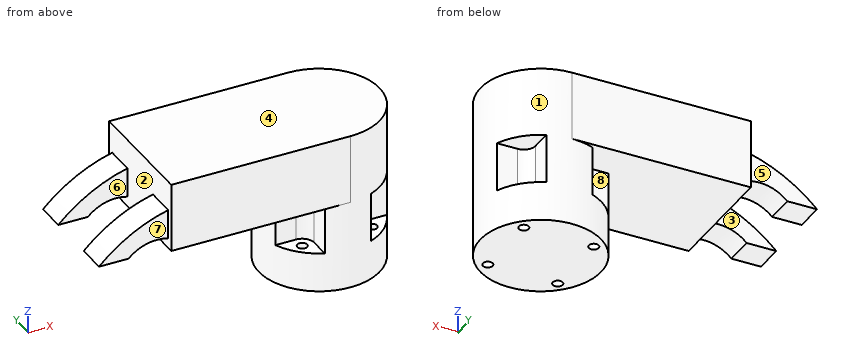
from build123d import *

# Parameters (mm, degrees)
SKETCH1_R                            = 30.5
BOSS_EXTRUDE1_DEPTH                  = 80
CUT_EXTRUDE1_REACH                   = 142.887
CUT_EXTRUDE1_START                   = -50
SKETCH2_R                            = 2.5
SKETCH7_W                            = 35
SKETCH7_H                            = 61
BOSS_EXTRUDE4_DEPTH                  = 60
BOSS_EXTRUDE4_DIRECTION_2_REACH      = 107.125
BOSS_EXTRUDE4_DIRECTION_2_END_RADIUS = 30.5
LOFT3_START                          = 12.5
LOFT3_DEPTH                          = 15
CUT_EXTRUDE2_START                   = -20
CUT_EXTRUDE2_DEPTH                   = 25
CIRPATTERN1_COUNT                    = 4


# Read off the part's stored shape, not the designer's step: Loft3
with BuildPart() as part:
    # Sketch1 → Boss-Extrude1 (new body)
    with BuildSketch(Plane.XY):
        Circle(SKETCH1_R)
    extrude(amount=BOSS_EXTRUDE1_DEPTH)

    # Sketch2 → Cut-Extrude1 (cut, up to next)
    with BuildSketch(Plane.XY.offset(80).offset(CUT_EXTRUDE1_START), mode=Mode.PRIVATE) as cut_extrude1_sk1:
        with Locations((17.68, -17.68)):
            Circle(SKETCH2_R)
    cut_extrude1_tool1 = extrude(cut_extrude1_sk1.sketch, amount=-CUT_EXTRUDE1_REACH, mode=Mode.PRIVATE) & part.part
    # Sketch2 → Cut-Extrude1 (cut, up to next)
    with BuildSketch(Plane.XY.offset(80).offset(CUT_EXTRUDE1_START), mode=Mode.PRIVATE) as cut_extrude1_sk2:
        with Locations((17.68, 17.68)):
            Circle(SKETCH2_R)
    cut_extrude1_tool2 = extrude(cut_extrude1_sk2.sketch, amount=-CUT_EXTRUDE1_REACH, mode=Mode.PRIVATE) & part.part
    # Sketch2 → Cut-Extrude1 (cut, up to next)
    with BuildSketch(Plane.XY.offset(80).offset(CUT_EXTRUDE1_START), mode=Mode.PRIVATE) as cut_extrude1_sk3:
        with Locations((-17.68, 17.68)):
            Circle(SKETCH2_R)
    cut_extrude1_tool3 = extrude(cut_extrude1_sk3.sketch, amount=-CUT_EXTRUDE1_REACH, mode=Mode.PRIVATE) & part.part
    # Sketch2 → Cut-Extrude1 (cut, up to next)
    with BuildSketch(Plane.XY.offset(80).offset(CUT_EXTRUDE1_START), mode=Mode.PRIVATE) as cut_extrude1_sk4:
        with Locations((-17.68, -17.68)):
            Circle(SKETCH2_R)
    cut_extrude1_tool4 = extrude(cut_extrude1_sk4.sketch, amount=-CUT_EXTRUDE1_REACH, mode=Mode.PRIVATE) & part.part
    add(cut_extrude1_tool1.solids().sort_by_distance((17.68, -17.68, 30))[0], mode=Mode.SUBTRACT)
    add(cut_extrude1_tool2.solids().sort_by_distance((17.68, 17.68, 30))[0], mode=Mode.SUBTRACT)
    add(cut_extrude1_tool3.solids().sort_by_distance((-17.68, 17.68, 30))[0], mode=Mode.SUBTRACT)
    add(cut_extrude1_tool4.solids().sort_by_distance((-17.68, -17.68, 30))[0], mode=Mode.SUBTRACT)

    # Sketch7 → Boss-Extrude4 (add)
    with BuildSketch(Plane.ZY.offset(30.5)):
        with Locations((62.5, 0)):
            Rectangle(SKETCH7_W, SKETCH7_H)
    extrude(amount=BOSS_EXTRUDE4_DEPTH)

    # Boss-Extrude4 direction 2: up to this cylinder (the profile starts outside it)
    boss_extrude4_direction_2_end = Plane(origin=(0, 0, 62.5), z_dir=(0, 0, -1)) * Cylinder(BOSS_EXTRUDE4_DIRECTION_2_END_RADIUS, 276.25, mode=Mode.PRIVATE)
    # Sketch7 → Boss-Extrude4 direction 2 (add, up to the surface)
    with BuildSketch(Plane.ZY.offset(30.5), mode=Mode.PRIVATE) as boss_extrude4_direction_2_sk1:
        with Locations((62.5, 0)):
            Rectangle(SKETCH7_W, SKETCH7_H)
    boss_extrude4_direction_2_tool1 = extrude(boss_extrude4_direction_2_sk1.sketch, amount=-BOSS_EXTRUDE4_DIRECTION_2_REACH, mode=Mode.PRIVATE) - boss_extrude4_direction_2_end
    add(boss_extrude4_direction_2_tool1.solids().sort_by_distance((-30.5, 0, 62.5))[0])
    add(boss_extrude4_direction_2_tool1.solids().sort_by_distance((-30.5, 0, 62.5))[1])

    # Loft3 outline → Loft3 (add)
    with BuildSketch(Plane(origin=(0, 0, 0), x_dir=(1, 0, 0), z_dir=(0, 1, 0)).offset(LOFT3_START)):
        with BuildLine():
            add(Edge.make_bspline(
                [(-90.5, -65), (-102.577141217, -62.16196551), (-115.272859166, -55.238036023), (-125.5, -45)],
                knots=[0, 0, 0, 0, 1, 1, 1, 1], degree=3))
            Line((-90.5, -65), (-90.5, -50))
            add(Edge.make_bspline(
                [(-90.5, -50), (-97.577141217, -52.16196551), (-105.272859166, -50.238036023), (-110.5, -45)],
                knots=[0, 0, 0, 0, 1, 1, 1, 1], degree=3))
            Line((-110.5, -45), (-125.5, -45))
        make_face()
    loft3 = extrude(amount=LOFT3_DEPTH)

    # Mirror1: Loft3 across plane
    add(loft3.mirror(Plane.ZX))

    # Sketch10 → Cut-Extrude2 (cut)
    with BuildSketch(Plane(origin=(0, 0, 0), x_dir=(-1, 0, 0), z_dir=(0, 0, -1)).offset(CUT_EXTRUDE2_START)):
        with BuildLine():
            Line((11.68, 17.68), (11.68, 28.174946318))
            ThreePointArc((11.68, 28.174946318), (21.566756826, 21.566756826), (28.174946318, 11.68))
            Line((28.174946318, 11.68), (17.68, 11.68))
            ThreePointArc((17.68, 11.68), (13.437359313, 13.437359313), (11.68, 17.68))
        make_face()
    cut_extrude2 = extrude(amount=-CUT_EXTRUDE2_DEPTH, mode=Mode.SUBTRACT)

    # CirPattern1: Cut-Extrude2 ×4 about axis
    cirpattern1_axis = Axis((0, 0, 0), (0, 0, 1))
    for i in range(1, CIRPATTERN1_COUNT):
        add(cut_extrude2.rotate(cirpattern1_axis, i * 360 / CIRPATTERN1_COUNT), mode=Mode.SUBTRACT)


solid = part.part
The model under review builds one solid part; all positions refer to its coordinate system, in mm. Face numbers are marked on the shaded views. A direction names the side the tool comes from. Give positions to 0.01 mm unless a question says otherwise; leave off trailing zeros. Write each loop counter-clockwise with the first axis right and the second up, starting at its lowest first coordinate (ties: lowest second). Pieces come first, ordered by that corner, then holes.
1. For P1, Ø3, axis at x = -25, z = 37, coming from the +Y side; P2, Ø17.5, axis at y = 5, z = 71, coming from the -X side; P3, Ø5, axis at y = 7, z = 48.5, coming from the +X side, all flat-tipped, find the tip position at first contact; note any pin that passes through.
2. Wall thickness on L1, parallel to Y at x = 17, z = 13; L2, parallel to Y at x = 17.68, z = 13.5; L3, parallel to Z at x = -77, y = -6: over which ranges is each line inside the solid? List them lowest first.
3. Draft analysis for pull direction Y (two halves, no side actions). For the marked faces 1, 2, 3 and 4, state which applies: +Y half, -Y half, draft (parallel to the pull), parting line (faces both ways), or undercut.
4. Tool access review of the marked faces 5, 6, 7 and 8: name each direction out of +Z, -Z, +X, -X, +Y, -Y from which nothing blocks a thin tool from reaching the whole face with its end or side.
5. Add section B-B, the plane y = 0. Write out the cut boundary in (x, z), plus the area to 3 significant figures.
6. Add section D-D, the plane z = 71. Write out the cut boundary in (x, y).
7. Add section A-A, the plane z = 23. Write out the cut boundary in (x, y).
8. Add section C-C, the plane x = -87. Write out the cut boundary in (y, z).
Worked answers:
1. P1: stops at y = 11.68
1. P2: stops at x = -90.5
1. P3: stops at x = 30.17
2. L1: y = -25.32 to -20.09, -15.27 to 15.27, 20.09 to 25.32
2. L2: y = -24.85 to -20.18, -15.18 to 15.18, 20.18 to 24.85
2. L3: z = 45 to 80
3. face 1: parting line
3. face 2: undercut
3. face 3: undercut
3. face 4: draft
4. face 5: +Z, -Z, -X, +Y
4. face 6: +Z, -Z, -X
4. face 7: +Z, -Z, -X, -Y
4. face 8: -X, +Y
5. outline: (-90.5, 45) - (-30.5, 45) - (-30.5, 0) - (30.5, 0) - (30.5, 80) - (-90.5, 80) - close
5. area: 6,980 mm2
6. outline: (-90.5, -30.5) - (0, -30.5) arc R30.5 ccw to (0, 30.5) - (-90.5, 30.5) - close
7. outline: (-28.17, -11.68) - (-17.68, -11.68) arc R6 cw to (-11.68, -17.68) - (-11.68, -28.17) arc R30.5 ccw to (11.68, -28.17) - (11.68, -17.68) arc R6 cw to (17.68, -11.68) - (28.17, -11.68) arc R30.5 ccw to (28.17, 11.68) - (17.68, 11.68) arc R6 cw to (11.68, 17.68) - (11.68, 28.17) arc R30.5 ccw to (-11.68, 28.17) - (-11.68, 17.68) arc R6 cw to (-17.68, 11.68) - (-28.17, 11.68) arc R30.5 ccw to start
8. outline: (-30.5, 45) - (30.5, 45) - (30.5, 80) - (-30.5, 80) - close
